from build123d import *

# Parameters (mm, degrees)
SKETCH1_W                                       = 15.24
SKETCH1_H                                       = 19.05
BOSS_EXTRUDE1_DEPTH                             = 25.4
BOSS_EXTRUDE5_DEPTH                             = 3.81
LPATTERN2_COUNT                                 = 2
LPATTERN2_PITCH                                 = 11.43
SKETCH10_R                                      = 1.905
CUT_EXTRUDE1_DEPTH                              = 16.24
BOSS_EXTRUDE6_DEPTH                             = 19.05
CUT_EXTRUDE2_DEPTH                              = 3.81
CBORE_FOR_6_PAN_HEAD_MACHINE_SCREW1_D           = 3.7500052
CBORE_FOR_6_PAN_HEAD_MACHINE_SCREW1_CBORE_D     = 7.5000104
CBORE_FOR_6_PAN_HEAD_MACHINE_SCREW1_CBORE_DEPTH = 2.032
CUT_EXTRUDE3_REACH                              = 15.208
SKETCH22_R                                      = 2.499995
FILLET1_R                                       = 0.5
FILLET2_R                                       = 0.5
CUT_EXTRUDE4_DEPTH                              = 1.27
CUT_EXTRUDE6_DEPTH                              = 3.048
FILLET3_R                                       = 0.5
CUT_EXTRUDE7_DEPTH                              = 1.27
SKETCH27_R                                      = 1.397
CUT_EXTRUDE8_DEPTH                              = 1.27


with BuildPart() as part:
    # Sketch1 → Boss-Extrude1 (new body)
    with BuildSketch(Plane.XY):
        Rectangle(SKETCH1_W, SKETCH1_H)
    extrude(amount=BOSS_EXTRUDE1_DEPTH)

    # Sketch9 → Boss-Extrude5 (add)
    with BuildSketch(Plane(origin=(7.62, 0, 0), x_dir=(0, 0, -1), z_dir=(1, 0, 0))):
        with BuildLine():
            Line((0, 9.525), (0, -9.525))
            ThreePointArc((0, -9.525), (8.798459024, 0), (0, 9.525))
        make_face()
    boss_extrude5 = extrude(amount=-BOSS_EXTRUDE5_DEPTH)

    # LPattern2: Boss-Extrude5 ×2
    with Locations(*[(-i * LPATTERN2_PITCH, 0, 0) for i in range(1, LPATTERN2_COUNT)]):
        add(boss_extrude5)

    # Sketch10 → Cut-Extrude1 (cut, through all)
    with BuildSketch(Plane(origin=(7.62, 0, 0), x_dir=(0, 0, -1), z_dir=(1, 0, 0))):
        with Locations((1.178459024, 0)):
            Circle(SKETCH10_R)
    extrude(amount=-CUT_EXTRUDE1_DEPTH, mode=Mode.SUBTRACT)

    # Sketch13 → Boss-Extrude6 (add)
    with BuildSketch(Plane(origin=(0, -9.525, 0), x_dir=(-1, 0, 0), z_dir=(0, -1, 0))):
        with BuildLine():
            Line((7.62, -25.4), (-7.62, -25.4))
            ThreePointArc((-7.62, -25.4), (0, -33.02), (7.62, -25.4))
        make_face()
    extrude(amount=-BOSS_EXTRUDE6_DEPTH)

    # Sketch17 → Cut-Extrude2 (cut, symmetric)
    with BuildSketch(Plane(origin=(0, 0, 0), x_dir=(0, 0, -1), z_dir=(1, 0, 0))):
        with BuildLine():
            Line((0, 9.525), (0, -9.525))
            ThreePointArc((0, -9.525), (-10.311535776, 0), (0, 9.525))
        make_face()
    extrude(amount=CUT_EXTRUDE2_DEPTH, both=True, mode=Mode.SUBTRACT)

    # CBORE for #6 Pan Head Machine Screw1 (through all)
    with Locations(Plane.ZY.offset(7.62)):
        with Locations((-1.178459024, 0)):
            CounterBoreHole(CBORE_FOR_6_PAN_HEAD_MACHINE_SCREW1_D / 2, CBORE_FOR_6_PAN_HEAD_MACHINE_SCREW1_CBORE_D / 2, CBORE_FOR_6_PAN_HEAD_MACHINE_SCREW1_CBORE_DEPTH)

    # Sketch22 → Cut-Extrude3 (cut, up to next)
    with BuildSketch(Plane.ZY.offset(5.588), mode=Mode.PRIVATE) as cut_extrude3_sk1:
        with Locations((-1.178459024, 0)):
            Circle(SKETCH22_R)
    cut_extrude3_tool1 = extrude(cut_extrude3_sk1.sketch, amount=-CUT_EXTRUDE3_REACH, mode=Mode.PRIVATE) & part.part
    add(cut_extrude3_tool1.solids().sort_by_distance((-5.588, 0, -1.178459))[0], mode=Mode.SUBTRACT)

    # Fillet1
    fillet1_edges = [part.edges().sort_by_distance(p)[0] for p in [
        (0, 9.525, 1.513076752),
        (0, -9.525, 1.513076752),
    ]]
    fillet(fillet1_edges, radius=FILLET1_R)

    # Fillet2
    fillet2_edges = [part.edges().sort_by_distance(p)[0] for p in [
        (-7.62, 0, -4.928464224),
        (-5.588, 0, -4.928464224),
    ]]
    fillet(fillet2_edges, radius=FILLET2_R)

    # Sketch18 → Cut-Extrude4 (cut)
    with BuildSketch(Plane(origin=(0, -9.525, 0), x_dir=(-1, 0, 0), z_dir=(0, -1, 0))):
        with BuildLine():
            Line((3.044880057, -17.007076752), (6.854880057, -17.007076752))
            ThreePointArc((6.854880057, -17.007076752), (6.332307247, -16.11715703), (6.858, -15.229076752))
            Line((6.858, -15.229076752), (1.778, -15.229076752))
            Line((1.778, -15.229076752), (1.778, -1.513076752))
            ThreePointArc((1.778, -1.513076752), (0, -3.291076752), (-1.778, -1.513076752))
            Line((-1.778, -1.513076752), (-1.778, -15.229076752))
            Line((-1.778, -15.229076752), (-6.858, -15.229076752))
            ThreePointArc((-6.858, -15.229076752), (-6.111619184, -16.118076752), (-6.858, -17.007076752))
            Line((-6.858, -17.007076752), (-3.048, -17.007076752))
            ThreePointArc((-3.048, -17.007076752), (-5.392804187, -22.012637101), (-5.614223517, -27.535744431))
            ThreePointArc((-5.614223517, -27.535744431), (-0.211295876, -32.163939746), (5.357263796, -27.736416493))
            ThreePointArc((5.357263796, -27.736416493), (5.298057191, -22.135324722), (3.044880057, -17.007076752))
        make_face()
    extrude(amount=-CUT_EXTRUDE4_DEPTH, mode=Mode.SUBTRACT)

    # Sketch23 → Cut-Extrude6 (cut)
    with BuildSketch(Plane.XZ.offset(9.525)):
        with BuildLine():
            Line((0, 19.008349223), (-3.846708267, 27.023019242))
            ThreePointArc((-3.846708267, 27.023019242), (-0.048818705, 29.690299102), (3.773291733, 27.057844207))
            Line((3.773291733, 27.057844207), (0, 19.008349223))
        make_face()
    extrude(amount=-CUT_EXTRUDE6_DEPTH, mode=Mode.SUBTRACT)

    # Fillet3
    fillet3_edges = [part.edges().sort_by_distance(p)[0] for p in [
        (0, -8.255, 5.568289649),
    ]]
    fillet(fillet3_edges, radius=FILLET3_R)

    # Sketch26 → Cut-Extrude7 (cut)
    with BuildSketch(Plane(origin=(0, -6.477, 0), x_dir=(-1, 0, 0), z_dir=(0, -1, 0))):
        with BuildLine():
            ThreePointArc((2.342289249, -26.290868459), (0.056289249, -28.576868459), (-2.229710751, -26.290868459))
            ThreePointArc((-2.229710751, -26.290868459), (0.056289249, -25.258930958), (2.342289249, -26.290868459))
        make_face()
    extrude(amount=-CUT_EXTRUDE7_DEPTH, mode=Mode.SUBTRACT)

    # Sketch27 → Cut-Extrude8 (cut)
    with BuildSketch(Plane.XZ.offset(5.207)):
        with Locations(Location((-0.056289249, 26.290868459, 0), (0, 0, 270))):  # turned: the seam where the file's is
            Circle(SKETCH27_R)
    extrude(amount=-CUT_EXTRUDE8_DEPTH, mode=Mode.SUBTRACT)


solid = part.part
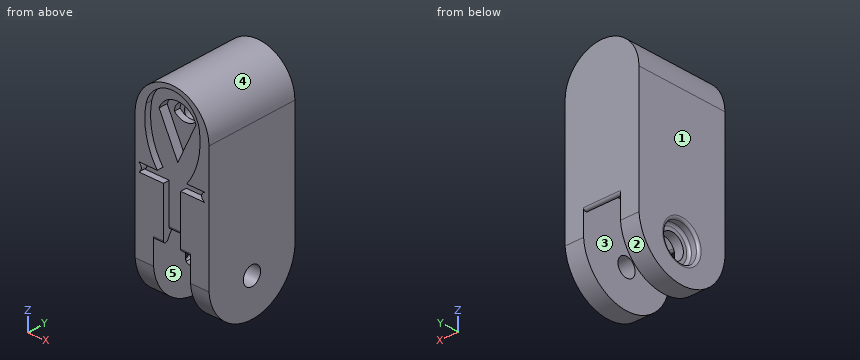
Can you work these out from the model? Positions are in its coordinate system, mm. Face numbers are marked on the shaded views. A direction names the side the tool comes from. Give positions to 0.01 mm unless a question says otherwise; leave off trailing zeros. Write each loop counter-clockwise with the first axis right and the second up, starting at its lowest first coordinate (ties: lowest second). Pieces come first, ordered by that corner, then holes. Notation, with made-up numbers: M 28.25,85 L 54.25,85 A21 cw 54.25,90 Z; hole C -1.75,-28 d1. An arc over 180 degrees is marked long. Answer in a Markdown table with one row per item. Add a question column.
Item 1: We'd pull the mould along X, two halves only. Please class the marked faces 1, 2 and 3: released by +X, released by -X, zero draft, split by the parting line, or undercut.
Item 2: Imagine slicing it at D-D, the plane y = 7.5. Write out the boundary of the cut face in (x, z).
Item 3: Imagine slicing it at A-A, the plane y = 0. Write out the boundary of the cut face in (x, z).
Item 4: On a 3-axis mill with a long thin cutter (end or side, diameter ignored), from which of +Z, -Z, +X, -X, +Y, -Y can I reach the whole of each face in a straight line? I mean the marked faces 4 and 5. Say none if no direction works.
Item 5: Please list where these lines run through material, in increasing order: L1, parallel to X at y = -3.5, z = 6.5; L2, parallel to Y at x = 0.5, z = 15.5 (3 decimals); L3, parallel to Z at x = 6.25, y = -0.75.
Item 6: For pin 1 Ø8 at (x, z) = (3, 3) entering from +Y (3 decimals); pin 2 Ø8 at (x, y) = (-5.5, -4.5) entering from -Z; pin 3 Ø1.4 at (x, y) = (-3.5, -9) entering from +Z; pin 4 Ø6 at (x, y) = (5, 6.5) entering from -Z, each with a flat end and sliding along its axis, tell me the tip position at first contact or that it passes through.
Item 7: Imagine slicing it at B-B, the plane x = -4.5. Write out the boundary of the cut face in (y, z) (3 decimals), plus the area to 3 significant figures.
Item 8: Imagine slicing it at C-C, the plane z = 23.5. Write out the boundary of the cut face in (x, y) (3 decimals).
Evaluation:
| question | item | result |
|---|---|---|
| 1 | face 1 | released by -X |
| 1 | face 2 | zero draft |
| 1 | face 3 | undercut |
| 2 | outline | M -7.62,-5.16 L -3.81,-5.16 L -3.81,6.68 L 3.81,6.68 L 3.81,-5.16 L 7.62,-5.16 L 7.62,25.4 A7.62 ccw -7.62,25.4 Z |
| 3 | outline | M -7.62,-8.8 L -3.81,-8.8 L -3.81,-3.68 L -5.59,-3.68 L -5.59,-4.43 A0.5 cw -6.09,-4.93 L -7.12,-4.93 A0.5 ccw -7.62,-5.43 Z; M -7.62,3.07 A0.5 ccw -7.12,2.57 L -6.09,2.57 A0.5 cw -5.59,2.07 L -5.59,1.32 L -3.81,1.32 L -3.81,10.31 L 3.81,10.31 L 3.81,0.73 L 7.62,0.73 L 7.62,25.4 A7.62 ccw -7.62,25.4 Z; M 3.81,-8.8 L 7.62,-8.8 L 7.62,-3.08 L 3.81,-3.08 Z |
| 4 | face 4 | +Z, +Y, -Y |
| 4 | face 5 | -Z |
| 5 | L1 | x = -7.62 to -3.81, 3.81 to 7.62 |
| 5 | L2 | y = -8.255 to 9.525 |
| 5 | L3 | z = -8.77 to -2.93, 0.57 to 29.76 |
| 6 | pin 1 | stops at y = 9.525 |
| 6 | pin 2 | stops at z = -8.79 |
| 6 | pin 3 | stops at z = 32.49 |
| 6 | pin 4 | stops at z = -8.13 |
| 7 | outline | M -9.525,0 A9.555 ccw 9.525,0 L 9.525,31.549 L -9.525,31.549 L -9.525,29.736 L -8.255,29.736 L -8.255,19.617 L -9.525,19.617 L -9.525,17.007 L -8.255,17.007 L -8.255,15.229 L -9.525,15.229 Z; hole C 0,-1.178 d5 |
| 7 | area | 695 mm² |
| 8 | outline | M -7.62,-9.525 L -5.522,-9.525 L -5.522,-8.255 L -2.156,-8.255 L -2.156,-6.477 L 2.106,-6.477 L 2.106,-8.255 L 5.671,-8.255 L 5.671,-9.525 L 7.62,-9.525 L 7.62,9.525 L -7.62,9.525 Z |
